Design review of the part shown in the three views and the two pictorial views. Dimensions are in mm from the part's minimum x, y and z. A direction names the side the tool comes from. Coordinates: 2 decimals unless noted, no trailing zeros. Loops run counter-clockwise (first coordinate to the right, second up) from the corner with the lowest first, then second, coordinate; pieces in that order, holes last.
Q1. Add section D-D on z = 26. Give the boundary of the cut face in (x, y), and give its area (3 significant figures).
Q2. Draft analysis for pull direction X (two halves, no side actions). For the marked faces 4, 5 and 6, state which applies: released by +X, released by -X, zero draft, split by the parting line, or undercut.
Q3. Machinability: for the marked faces 1, 2 and 3, which of the approach directions +Z, -Z, +X, -X, +Y, -Y give a long, thin tool a straight path to every point of the face, cutting with its end or side? Answer none if there is none.
Q4. Add section C-C on y = 5. Give the boundary of the cut face in (x, z).
Q5. Add section A-A on x = 34. Give the boundary of the cut face in (y, z).
Q6. For P1, Ø8, axis at x = 36, z = 33.5, coming from the +Y side; P2, Ø10, axis at x = 29, y = 42, coming from the -Z side; P3, Ø1, axis at y = 34.5, z = 5.5, coming from the +X side, all flat-tipped, find the tip position at first contact; note any pin that passes through.
Q7. Wall thickness on probe 1 along X at (y, z) = (23, 12.5); probe 2 along Y at (x, z) = (34, 25); probe 3 along X at (y, z) = (15, 23): over which ranges is each line inside the solid? List them lowest first.
Q8. Add section B-B on z = 10. Give the boundary of the cut face in (x, y), and give its area (3 significant figures).
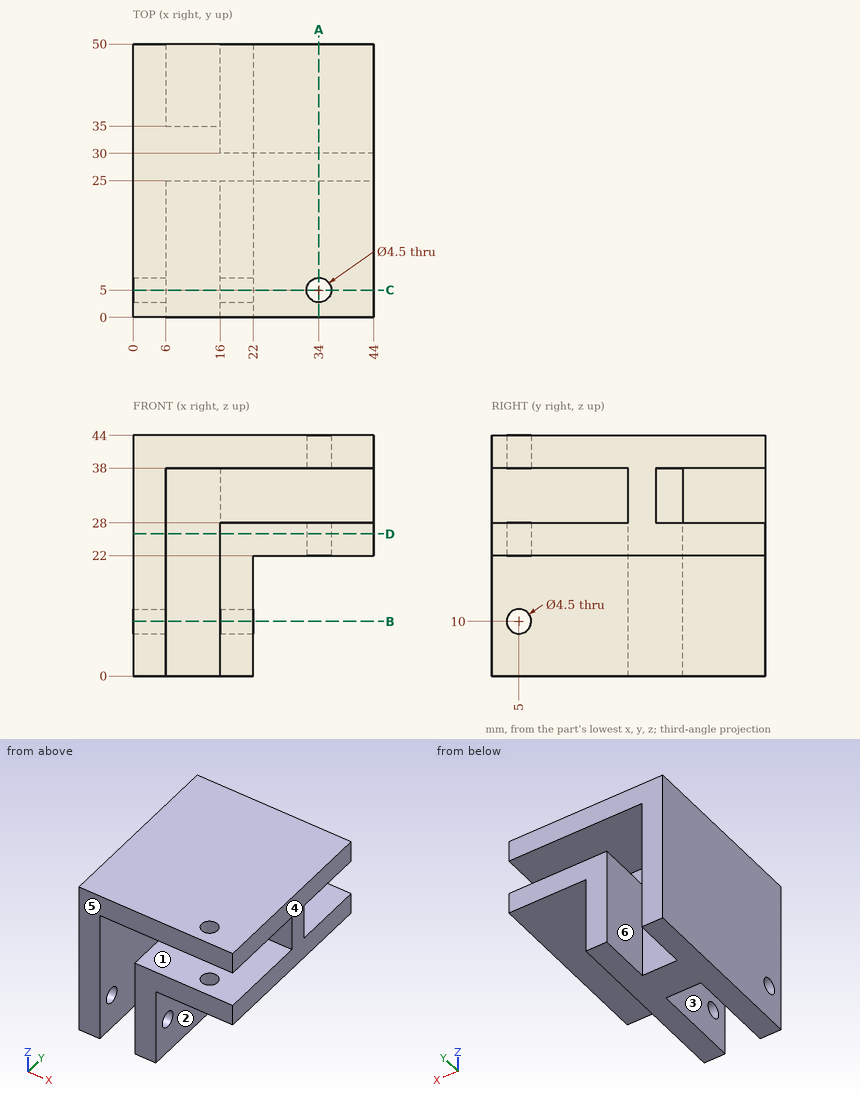
Entries:
1. outline: (0, 0) - (6, 0) - (6, 25) - (16, 25) - (16, 0) - (44, 0) - (44, 50) - (16, 50) - (16, 35) - (6, 35) - (6, 50) - (0, 50) - close; hole circle Ø4.5 at (34, 5)
1. area: 1,780 mm2
2. face 4: released by +X
2. face 5: zero draft
2. face 6: undercut
3. face 1: +X, -Y
3. face 2: -Z, +X, +Y, -Y
3. face 3: -Z, -Y
4. outline: (0, 0) - (6, 0) - (6, 7.75) - (0, 7.75) - close; (0, 12.25) - (6, 12.25) - (6, 38) - (31.75, 38) - (31.75, 44) - (0, 44) - close; (16, 0) - (22, 0) - (22, 7.75) - (16, 7.75) - close; (16, 12.25) - (22, 12.25) - (22, 22) - (31.75, 22) - (31.75, 28) - (16, 28) - close; (36.25, 22) - (44, 22) - (44, 28) - (36.25, 28) - close; (36.25, 38) - (44, 38) - (44, 44) - (36.25, 44) - close
5. outline: (0, 22) - (2.75, 22) - (2.75, 28) - (0, 28) - close; (0, 38) - (2.75, 38) - (2.75, 44) - (0, 44) - close; (7.25, 22) - (50, 22) - (50, 28) - (30, 28) - (30, 38) - (50, 38) - (50, 44) - (7.25, 44) - (7.25, 38) - (25, 38) - (25, 28) - (7.25, 28) - close
6. P1: stops at y = 30
6. P2: stops at z = 22
6. P3: stops at x = 22
7. probe 1: x = 0 to 6, 16 to 22
7. probe 2: y = 0 to 2.75, 7.25 to 50
7. probe 3: x = 0 to 6, 16 to 44
8. outline: (0, 0) - (6, 0) - (6, 2.75) - (0, 2.75) - close; (0, 7.25) - (6, 7.25) - (6, 25) - (16, 25) - (16, 7.25) - (22, 7.25) - (22, 50) - (16, 50) - (16, 35) - (6, 35) - (6, 50) - (0, 50) - close; (16, 0) - (22, 0) - (22, 2.75) - (16, 2.75) - close
8. area: 646 mm2
